CAD build for the part. Positions are in the model's coordinates, mm. A direction names the side the tool comes from. Round coordinates to 2 decimals unless told otherwise and drop trailing zeros. Loops run counter-clockwise (first coordinate to the right, second up) from the corner with the lowest first, then second, coordinate; pieces in that order, holes last.
from build123d import *

# Parameters (mm, degrees)
BOSS_EXTRUDE1_DEPTH = 5
CIRPATTERN4_COUNT   = 20
SKETCH6_R           = 8.75
BOSS_EXTRUDE2_DEPTH = 5


with BuildPart() as part:
    # Sketch3 → Boss-Extrude1 (new body)
    with BuildSketch(Plane(origin=(0, 0, 0), x_dir=(1, 0, 0), z_dir=(0, 1, 0))):
        with BuildLine():
            Line((1.629672464, 9.254533474), (1.517478561, 8.617410215))
            ThreePointArc((1.517478561, 8.617410215), (0.761630034, 8.716789529), (0, 8.75))
            Line((0, 8.75), (0, 9.396926208))
            ThreePointArc((0, 9.396926208), (0.25763458, 10.219055101), (0.661482168, 10.980092957))
            ThreePointArc((0.661482168, 10.980092957), (0.957477757, 10.958249694), (1.252776281, 10.928428597))
            ThreePointArc((1.252776281, 10.928428597), (1.518520476, 10.108885116), (1.629672464, 9.254533474))
        make_face()
    extrude(amount=BOSS_EXTRUDE1_DEPTH)


with BuildPart() as cirpattern4_1:
    # CirPattern4: pattern copy
    add(part.part.rotate(Axis((0, 0, 0), (0, 1, 0)), 1 * 360 / CIRPATTERN4_COUNT))


with BuildPart() as cirpattern4_2:
    # CirPattern4: pattern copy
    add(part.part.rotate(Axis((0, 0, 0), (0, 1, 0)), 2 * 360 / CIRPATTERN4_COUNT))


with BuildPart() as cirpattern4_3:
    # CirPattern4: pattern copy
    add(part.part.rotate(Axis((0, 0, 0), (0, 1, 0)), 3 * 360 / CIRPATTERN4_COUNT))


with BuildPart() as cirpattern4_4:
    # CirPattern4: pattern copy
    add(part.part.rotate(Axis((0, 0, 0), (0, 1, 0)), 4 * 360 / CIRPATTERN4_COUNT))


with BuildPart() as cirpattern4_5:
    # CirPattern4: pattern copy
    add(part.part.rotate(Axis((0, 0, 0), (0, 1, 0)), 5 * 360 / CIRPATTERN4_COUNT))


with BuildPart() as cirpattern4_6:
    # CirPattern4: pattern copy
    add(part.part.rotate(Axis((0, 0, 0), (0, 1, 0)), 6 * 360 / CIRPATTERN4_COUNT))


with BuildPart() as cirpattern4_7:
    # CirPattern4: pattern copy
    add(part.part.rotate(Axis((0, 0, 0), (0, 1, 0)), 7 * 360 / CIRPATTERN4_COUNT))


with BuildPart() as cirpattern4_8:
    # CirPattern4: pattern copy
    add(part.part.rotate(Axis((0, 0, 0), (0, 1, 0)), 8 * 360 / CIRPATTERN4_COUNT))


with BuildPart() as cirpattern4_9:
    # CirPattern4: pattern copy
    add(part.part.rotate(Axis((0, 0, 0), (0, 1, 0)), 9 * 360 / CIRPATTERN4_COUNT))


with BuildPart() as cirpattern4_10:
    # CirPattern4: pattern copy
    add(part.part.rotate(Axis((0, 0, 0), (0, 1, 0)), 10 * 360 / CIRPATTERN4_COUNT))


with BuildPart() as cirpattern4_11:
    # CirPattern4: pattern copy
    add(part.part.rotate(Axis((0, 0, 0), (0, 1, 0)), 11 * 360 / CIRPATTERN4_COUNT))


with BuildPart() as cirpattern4_12:
    # CirPattern4: pattern copy
    add(part.part.rotate(Axis((0, 0, 0), (0, 1, 0)), 12 * 360 / CIRPATTERN4_COUNT))


with BuildPart() as cirpattern4_13:
    # CirPattern4: pattern copy
    add(part.part.rotate(Axis((0, 0, 0), (0, 1, 0)), 13 * 360 / CIRPATTERN4_COUNT))


with BuildPart() as cirpattern4_14:
    # CirPattern4: pattern copy
    add(part.part.rotate(Axis((0, 0, 0), (0, 1, 0)), 14 * 360 / CIRPATTERN4_COUNT))


with BuildPart() as cirpattern4_15:
    # CirPattern4: pattern copy
    add(part.part.rotate(Axis((0, 0, 0), (0, 1, 0)), 15 * 360 / CIRPATTERN4_COUNT))


with BuildPart() as cirpattern4_16:
    # CirPattern4: pattern copy
    add(part.part.rotate(Axis((0, 0, 0), (0, 1, 0)), 16 * 360 / CIRPATTERN4_COUNT))


with BuildPart() as cirpattern4_17:
    # CirPattern4: pattern copy
    add(part.part.rotate(Axis((0, 0, 0), (0, 1, 0)), 17 * 360 / CIRPATTERN4_COUNT))


with BuildPart() as cirpattern4_18:
    # CirPattern4: pattern copy
    add(part.part.rotate(Axis((0, 0, 0), (0, 1, 0)), 18 * 360 / CIRPATTERN4_COUNT))


with BuildPart() as cirpattern4_19:
    # CirPattern4: pattern copy
    add(part.part.rotate(Axis((0, 0, 0), (0, 1, 0)), 19 * 360 / CIRPATTERN4_COUNT))


with BuildPart() as part_1:
    add(part.part)

    add(cirpattern4_1.part)  # Boss-Extrude2 merges CirPattern4_1

    add(cirpattern4_2.part)  # Boss-Extrude2 merges CirPattern4_2

    add(cirpattern4_3.part)  # Boss-Extrude2 merges CirPattern4_3

    add(cirpattern4_4.part)  # Boss-Extrude2 merges CirPattern4_4

    add(cirpattern4_5.part)  # Boss-Extrude2 merges CirPattern4_5

    add(cirpattern4_6.part)  # Boss-Extrude2 merges CirPattern4_6

    add(cirpattern4_7.part)  # Boss-Extrude2 merges CirPattern4_7

    add(cirpattern4_8.part)  # Boss-Extrude2 merges CirPattern4_8

    add(cirpattern4_9.part)  # Boss-Extrude2 merges CirPattern4_9

    add(cirpattern4_10.part)  # Boss-Extrude2 merges CirPattern4_10

    add(cirpattern4_11.part)  # Boss-Extrude2 merges CirPattern4_11

    add(cirpattern4_12.part)  # Boss-Extrude2 merges CirPattern4_12

    add(cirpattern4_13.part)  # Boss-Extrude2 merges CirPattern4_13

    add(cirpattern4_14.part)  # Boss-Extrude2 merges CirPattern4_14

    add(cirpattern4_15.part)  # Boss-Extrude2 merges CirPattern4_15

    add(cirpattern4_16.part)  # Boss-Extrude2 merges CirPattern4_16

    add(cirpattern4_17.part)  # Boss-Extrude2 merges CirPattern4_17

    add(cirpattern4_18.part)  # Boss-Extrude2 merges CirPattern4_18

    add(cirpattern4_19.part)  # Boss-Extrude2 merges CirPattern4_19
    # Sketch6 → Boss-Extrude2 (add)
    with BuildSketch(Plane(origin=(0, 0, 0), x_dir=(1, 0, 0), z_dir=(0, 1, 0))):
        Circle(SKETCH6_R)
    extrude(amount=BOSS_EXTRUDE2_DEPTH)


solid = part_1.part
Item 1: Mould opens along Z. For faces 6 (the cylindrical face through (1.516, 2.465, -10.121)), 7 (the flat face through (0, 5, 0)), 8 (the cylindrical face through (2.914, 2.465, 9.786)) say: released by +Z, released by -Z, zero draft, split by the parting line, or undercut.
Verdict:
face 6: released by -Z
face 7: zero draft
face 8: undercut
Item 2: 3-axis set-ups, long thin cutter, end or side, ignore diameter. For faces 1 (the cylindrical face through (10.121, 2.465, 1.516)), 2 (the cylindrical face through (-6.205, 2.465, 8.11)), 3 (the cylindrical face through (0.253, 2.465, -10.208)), 4 (the cylindrical face through (-9.63, 2.465, -3.395)), 5 (the cylindrical face through (5.619, 2.465, 6.708)): which of +Z, -Z, +X, -X, +Y, -Y reach the whole face in a straight line?
Verdict:
face 1: +X, +Y, -Y
face 2: +Z, +Y, -Y
face 3: -Z, +Y, -Y
face 4: -X, +Y, -Y
face 5: +Y, -Y
Item 3: Wall check: L1, parallel to X at y = 3.65, z = 7.75; L2, parallel to Z at x = 6.25, y = 2; L3, parallel to X at y = 3.85, z = -7.75. Give the ranges that are in metal, low to high.
Verdict:
L1: x = -7.34 to -5.7, -4.12 to 5.59
L2: z = -8.14 to 6.47
L3: x = -5.59 to 4.12, 5.7 to 7.34
Item 4: Cut at A-A (x = 3.5). List the corners of the cut face in (y, z).
Verdict:
outline: (0, -9.75) - (5, -9.75) - (5, 8.02) - (0, 8.02) - close
Item 5: Flat gauge pins, fed straight in: P1, Ø2, axis at x = 4.5, y = 3.5, coming from the +Z side; P2, Ø0.5, axis at x = 9, y = 3, coming from the -Z side; P3, Ø1, axis at x = -8, z = -8.5, coming from the -Y side (3 decimals). Where does each tip first touch, or does it go through?
Verdict:
P1: stops at z = 9.58
P2: stops at z = -5.92
P3: passes through
